from build123d import *

# Parameters (mm, degrees)
BOSS_EXTRUDE1_DEPTH        = 7.62
CUT_EXTRUDE1_DEPTH         = 30.441514138
SKETCH3_W                  = 12.7
SKETCH3_H                  = 7.62
M2_5_CLEARANCE_HOLE1_D     = 2.7051
M3_CLEARANCE_HOLE1_D       = 3.556
M3_CLEARANCE_HOLE1_DEPTH   = 5.08
M2_5_CLEARANCE_HOLE2_D     = 2.7051
M2_5_CLEARANCE_HOLE2_DEPTH = 15.375384182


with BuildPart() as part:
    # Sketch1 → Boss-Extrude1 (new body)
    with BuildSketch(Plane.XZ):
        with BuildLine():
            Line((17.227118157, -6.35), (23.057960451, -6.35))
            Line((23.057960451, -6.35), (23.057960451, 6.35))
            Line((23.057960451, 6.35), (17.227118157, 6.35))
            ThreePointArc((17.227118157, 6.35), (15.786457002, 6.695667846), (14.659490486, 7.657404449))
            ThreePointArc((14.659490486, 7.657404449), (14.589471792, 9.508848608), (15.564771332, 11.084138707))
            ThreePointArc((15.564771332, 11.084138707), (15.715448212, 15.715448212), (11.084138707, 15.564771332))
            ThreePointArc((11.084138707, 15.564771332), (9.317430783, 14.545190239), (7.295007228, 14.810907114))
            ThreePointArc((7.295007228, 14.810907114), (0, 16.51), (-7.295007228, 14.810907114))
            ThreePointArc((-7.295007228, 14.810907114), (-9.317430783, 14.545190239), (-11.084138707, 15.564771332))
            ThreePointArc((-11.084138707, 15.564771332), (-15.715448212, 15.715448212), (-15.564771332, 11.084138707))
            ThreePointArc((-15.564771332, 11.084138707), (-14.545190239, 9.317430783), (-14.810907114, 7.295007228))
            ThreePointArc((-14.810907114, 7.295007228), (-16.51, 0), (-14.810907114, -7.295007228))
            ThreePointArc((-14.810907114, -7.295007228), (-14.545190239, -9.317430783), (-15.564771332, -11.084138707))
            ThreePointArc((-15.564771332, -11.084138707), (-15.715448212, -15.715448212), (-11.084138707, -15.564771332))
            ThreePointArc((-11.084138707, -15.564771332), (-9.317430783, -14.545190239), (-7.295007228, -14.810907114))
            ThreePointArc((-7.295007228, -14.810907114), (0, -16.51), (7.295007228, -14.810907114))
            ThreePointArc((7.295007228, -14.810907114), (9.317430783, -14.545190239), (11.084138707, -15.564771332))
            ThreePointArc((11.084138707, -15.564771332), (15.715448212, -15.715448212), (15.564771332, -11.084138707))
            ThreePointArc((15.564771332, -11.084138707), (14.589471792, -9.508848608), (14.659490486, -7.657404449))
            ThreePointArc((14.659490486, -7.657404449), (15.786457002, -6.695667846), (17.227118157, -6.35))
        make_face()
    extrude(amount=-BOSS_EXTRUDE1_DEPTH)

    # Sketch2 → Cut-Extrude1 (cut, through all)
    with BuildSketch(Plane(origin=(0, 7.62, 0), x_dir=(-1, 0, 0), z_dir=(0, 1, 0))):
        with BuildLine():
            Line((-23.057960451, 1.27), (-23.057960451, -1.27))
            Line((-23.057960451, -1.27), (-12.636340451, -1.27))
            ThreePointArc((-12.636340451, -1.27), (-12.7, 0), (-12.636340451, 1.27))
            Line((-12.636340451, 1.27), (-23.057960451, 1.27))
        make_face()
    extrude(amount=-CUT_EXTRUDE1_DEPTH, mode=Mode.SUBTRACT)

    # Sketch3 → Cut-Revolve1 (revolve, cut)
    with BuildSketch(Plane.XY):
        with Locations((6.35, 3.81)):
            Rectangle(SKETCH3_W, SKETCH3_H)
    revolve(axis=Axis((0, 7.62, 0), (0, -1, 0)), mode=Mode.SUBTRACT)

    # M2.5 Clearance Hole1 (through all)
    with Locations(Plane(origin=(0, 0, 0), x_dir=(-1, 0, 0), z_dir=(0, -1, 0))):
        with Locations((-13.470384182, -13.470384182), (13.470384182, -13.470384182), (13.470384182, 13.470384182), (-13.470384182, 13.470384182)):
            Hole(M2_5_CLEARANCE_HOLE1_D / 2)

    # M3 Clearance Hole1
    with Locations(Plane.XY.offset(6.35)):
        with Locations((19.438793191, 3.81)):
            Hole(M3_CLEARANCE_HOLE1_D / 2, depth=M3_CLEARANCE_HOLE1_DEPTH)

    # M2.5 Clearance Hole2
    with Locations(Plane.XY.offset(-1.27)):
        with Locations((19.438793191, 3.81)):
            Hole(M2_5_CLEARANCE_HOLE2_D / 2, depth=M2_5_CLEARANCE_HOLE2_DEPTH)


solid = part.part
The listing builds one solid part. Answer for the finished solid, in the listing's coordinates (mm). A direction names the side the tool comes from. Give positions to 0.01 mm unless a question says otherwise; leave off trailing zeros. Write each loop counter-clockwise with the first axis right and the second up, starting at its lowest first coordinate (ties: lowest second). Pieces come first, ordered by that corner, then holes.
1) Section D-D (z = -3.5) is taken. Write down the section's boundary in (x, y), and give its area (3 significant figures).
2) Section C-C (y = 3.81) is taken. Count the separate pieces of the cut face and the enclosed holes in it, and give its area (3 significant figures).
3) Given P1, Ø1.6, axis at x = -13.47, z = 13.47, coming from the +Y side; P2, Ø3, axis at x = 19.44, y = 3.81, coming from the -Z side; P3, Ø1, axis at x = 8.5, y = 2.5, coming from the +Z side; P4, Ø1.5, axis at x = -8, y = 4, coming from the +Z side, each flat-ended and moving along its own axis, determine where each tip first touches the part or whether it passes through.
4) Find the intervals of material crossed by L1, parallel to X at y = 6.25, z = 13.5; L2, parallel to Z at x = 0, y = 5; L3, parallel to Z at x = -13, y = 0.75, in increasing order.
5) A tool of negligible diameter and unlimited length cuts with its end or side. For faces 5 (the face through (21.5, 3.8, 6.35)), 6 (the face through (15.768, 3.757, -6.705)), 7 (the face through (-16.51, 3.76, 0.11)), from which of +Z, -Z, +X, -X, +Y, -Y can it reach the whole face along a straight path? Write none if from no direction.
6) For a pull along Y with two mould halves and no side action, classify faces 1 (the face through (21, 5, -6.35)), 2 (the face through (7, 0, -11)), 3 (the face through (18.15, 4.22, -3.85)), 4 (the face through (17.74, 4.34, 3.77)) as pulls with the +Y half, pulls with the -Y half, needs draft (parallel to the pull), parting line crosses it, or undercut.
7) Section A-A (x = 0) is taken. Write down the section's boundary in (y, z).
8) Section B-B (z = 3.5) is taken. Write down the section's boundary in (x, y), and give its area (3 significant figures).
Response:
1. outline: (-16.13, 0) - (-12.21, 0) - (-12.21, 7.62) - (-16.13, 7.62) - close; (12.21, 0) - (23.06, 0) - (23.06, 7.62) - (12.21, 7.62) - close; hole circle Ø2.71 at (19.44, 3.81)
1. area: 107 mm2
2. separate pieces: 3
2. enclosed holes: 4
2. area: 497 mm2
3. P1: passes through
3. P2: stops at z = -6.35
3. P3: stops at z = 14.56
3. P4: stops at z = 14.83
4. L1: x = -16.65 to -14.82, -12.12 to 12.12, 14.82 to 16.65
4. L2: z = -16.51 to -12.7, 12.7 to 16.51
4. L3: z = -16.61 to -14.74, -12.2 to 12.2, 14.74 to 16.61
5. face 5: +Z, +X, +Y, -Y
5. face 6: +X, +Y, -Y
5. face 7: -X, +Y, -Y
6. face 1: needs draft
6. face 2: pulls with the -Y half
6. face 3: undercut
6. face 4: undercut
7. outline: (0, -16.51) - (7.62, -16.51) - (7.62, -12.7) - (0, -12.7) - close; (0, 12.7) - (7.62, 12.7) - (7.62, 16.51) - (0, 16.51) - close
8. outline: (-16.13, 0) - (-12.21, 0) - (-12.21, 7.62) - (-16.13, 7.62) - close; (12.21, 0) - (23.06, 0) - (23.06, 7.62) - (12.21, 7.62) - close; hole circle Ø3.56 at (19.44, 3.81)
8. area: 103 mm2
